```python
from build123d import *

# Parameters (mm, degrees)
F1_DEPTH = 57.15
F2_R     = 28.57499
F3_R     = 28.57499
F4_R     = 9.92251
F5_DEPTH = 88.901
F6_R     = 10.3251
F7_DEPTH = 7.9375


# Not quite as in the source:
# - a fillet or chamfer is up to 0.001 mm smaller than in the source, because OpenCascade refuses the exact size


with BuildPart() as f1:
    # F0 (on Front) → F1 (new body)
    with BuildSketch(Plane.XZ):
        with BuildLine():
            ThreePointArc((-44.45, 12.7), (-40.7302561211, 3.7197438789), (-31.75, 0))
            Line((-31.75, 0), (31.75, 0))
            ThreePointArc((31.75, 0), (40.7302561211, 3.7197438789), (44.45, 12.7))
            Line((44.45, 12.7), (44.45, 73.025))
            Line((44.45, 73.025), (36.5125, 73.025))
            Line((36.5125, 73.025), (36.5125, 12.7))
            ThreePointArc((36.5125, 12.7), (35.1175960454, 9.3324039546), (31.75, 7.9375))
            Line((31.75, 7.9375), (-31.75, 7.9375))
            ThreePointArc((-31.75, 7.9375), (-35.1175960454, 9.3324039546), (-36.5125, 12.7))
            Line((-36.5125, 12.7), (-36.5125, 73.025))
            Line((-36.5125, 73.025), (-44.45, 73.025))
            Line((-44.45, 73.025), (-44.45, 12.7))
        make_face()
    extrude(amount=-F1_DEPTH)

    # F2 (radius 28.575 in the source; OpenCascade refuses exactly that, so slightly less here)
    f2_edges = [f1.edges().sort_by_distance(p)[0] for p in [
        (40.48125, 0, 73.025),
        (40.48125, 57.15, 73.025),
    ]]
    fillet(f2_edges, radius=F2_R)

    # F3 (radius 28.575 in the source; OpenCascade refuses exactly that, so slightly less here)
    f3_edges = [f1.edges().sort_by_distance(p)[0] for p in [
        (-40.48125, 0, 73.025),
        (-40.48125, 57.15, 73.025),
    ]]
    fillet(f3_edges, radius=F3_R)

    # F4 (on face) → F5 (cut, through all)
    with BuildSketch(Plane(origin=(-44.45, 0, 0), x_dir=(0, -1, 0), z_dir=(-1, 0, 0))):
        with Locations((-29.956350103, 44.45)):
            Circle(F4_R)
    extrude(amount=-F5_DEPTH, mode=Mode.SUBTRACT)

    # F6 (on face) → F7 (join, through all)
    with BuildSketch(Plane.XY.offset(7.9375)):
        with BuildLine():
            Line((22.225, -53.975), (22.225, -6.35))
            ThreePointArc((22.225, -6.35), (24.0848719395, -1.8598719395), (28.575, 0))
            Line((28.575, 0), (-28.575, 0))
            ThreePointArc((-28.575, 0), (-24.0848719395, -1.8598719395), (-22.225, -6.35))
            Line((-22.225, -6.35), (-22.225, -53.975))
            ThreePointArc((-22.225, -53.975), (0, -76.2), (22.225, -53.975))
        make_face()
        with Locations((0, -53.975)):
            Circle(F6_R, mode=Mode.SUBTRACT)
        with Locations((0, -15.875)):
            Circle(F6_R, mode=Mode.SUBTRACT)
    extrude(amount=-F7_DEPTH)


solid = f1.part
```
Model file for the job. Use its own axes, mm. A direction names the side the tool comes from. Coordinates: 2 decimals unless noted, no trailing zeros. Order: outer loops, then holes, each group sorted by start corner. A loop starts at its lowest first (then second) coordinate and runs counter-clockwise, first axis right, second up. Notation, with made-up numbers: (66, 79) - (80, 79) arc R12 cw to (80, 90) - close; hole circle Ø1 at (82.5, 50). An arc over 180 degrees is marked (long way). Return JSON: item names as keys, results as strings. Group by question number.
1) Tool access for faces 5 (the cylindrical face through (-35.08, 28.175, 9.296)), 6 (the flat face through (-0.6, 57.15, 7.7)), 7 (the flat face through (38, 0, 23)): list every direction of +Z, -Z, +X, -X, +Y, -Y with a clear straight run to the whole face (end or side of a thin tool).
2) Probe line 1 (Y direction, x = 0, z = 2.5); line 2 (X direction, y = 38.5, z = 64.5); line 3 (Z direction, x = 6, y = -62.5). List the from-to ranges inside material, lowest first. Write a range as from..to.
3) Saw through at B-B, the plane x = 0. Write the cut outline in (y, z), plus the area to 3 significant figures.
4) Mould opens along Y. For faces 1 (the flat face through (-38, 0, 23)), 2 (the cylindrical face through (-41, 28, 4)), 3 (the cylindrical face through (40.426, 25.378, 35.647)), 4 (the cylindrical face through (5.6, -7.2, 4)) say: released by +Y, released by -Y, zero draft, split by the parting line, or undercut.
5) Saw through at D-D, the plane z = 40. Write the cut outline in (x, y), plus the area to 3 significant figures.
6) Saw through at A-A, the plane z = 17.5. Write the cut outline in (x, y).
7) Saw through at C-C, the plane y = -19. Write the cut outline in (x, z) (1 decimal), plus the area to 3 significant figures.
8) Flat gauge pins, fed straight in: P1, Ø10, axis at x = 18, z = 15, coming from the +Y side; P2, Ø4, axis at y = -24.5, z = 4, coming from the +X side (3 decimals); P3, Ø5, axis at x = -39.5, z = 21, coming from the -Y side; P4, Ø2.5, axis at y = -28, z = 5.5, coming from the -X side (3 decimals). Where does each tip first touch, or does it go through?
Values found:
{
 "1": {"face 5": "+Z, +Y, -Y", "face 6": "+Z, -Z, +X, -X, +Y", "face 7": "+Z, -Z, +X, -Y"},
 "2": {"line 1": "y = -76.2..-64.3, -43.65..-26.2, -5.55..57.15", "line 2": "x = -44.45..-36.51, 36.51..44.45", "line 3": "z = 0..7.94"},
 "3": {"outline": "(-76.2, 0) - (-64.3, 0) - (-64.3, 7.94) - (-76.2, 7.94) - close; (-43.65, 0) - (-26.2, 0) - (-26.2, 7.94) - (-43.65, 7.94) - close; (-5.55, 0) - (57.15, 0) - (57.15, 7.94) - (-5.55, 7.94) - close", "area": "731 mm²"},
 "4": {"face 1": "released by -Y", "face 2": "zero draft", "face 3": "undercut", "face 4": "undercut"},
 "5": {"outline": "(-44.45, 0) - (-36.51, 0) - (-36.51, 21.09) - (-44.45, 21.09) - close; (-44.45, 38.83) - (-36.51, 38.83) - (-36.51, 57.15) - (-44.45, 57.15) - close; (36.51, 0) - (44.45, 0) - (44.45, 21.09) - (36.51, 21.09) - close; (36.51, 38.83) - (44.45, 38.83) - (44.45, 57.15) - (36.51, 57.15) - close", "area": "626 mm²"},
 "6": {"outline": "(-44.45, 0) - (-36.51, 0) - (-36.51, 57.15) - (-44.45, 57.15) - close; (36.51, 0) - (44.45, 0) - (44.45, 57.15) - (36.51, 57.15) - close"},
 "7": {"outline": "(-22.2, 0) - (-9.8, 0) - (-9.8, 7.9) - (-22.2, 7.9) - close; (9.8, 0) - (22.2, 0) - (22.2, 7.9) - (9.8, 7.9) - close", "area": "197 mm²"},
 "8": {"P1": "passes through", "P2": "stops at x = 22.225", "P3": "stops at y = 0", "P4": "stops at x = -22.225"}
}
